```python
from build123d import *

# Parameters (mm, degrees)
SALIENTE_EXTRUIR1_DEPTH = 4
SALIENTE_EXTRUIR2_DEPTH = 30
SALIENTE_EXTRUIR5_DEPTH = 4
SALIENTE_EXTRUIR7_DEPTH = 4
CORTAR_EXTRUIR2_DEPTH   = 31
CROQUIS13_R             = 2.05
CORTAR_EXTRUIR3_DEPTH   = 4
CORTAR_EXTRUIR4_DEPTH   = 5
CORTAR_EXTRUIR5_DEPTH   = 2


with BuildPart() as part:
    # Croquis1 → Saliente-Extruir1 (new body)
    with BuildSketch(Plane(origin=(0, 0, 0), x_dir=(1, 0, 0), z_dir=(0, 1, 0))):
        Polygon((-11.66726189, 1.66726189), (11.66726189, -21.66726189), (11.66726189, 21.66726189), (-11.66726189, 21.66726189), align=None)
    extrude(amount=SALIENTE_EXTRUIR1_DEPTH)

    # Croquis3 → Saliente-Extruir2 (add)
    with BuildSketch(Plane.XZ):
        Polygon((-11.66726189, -1.66726189), (-11.66726189, 3.98959236), (11.66726189, 27.324116139), (11.66726189, 21.66726189), align=None)
    extrude(amount=-SALIENTE_EXTRUIR2_DEPTH)

    # Croquis7 → Saliente-Extruir5 (add)
    with BuildSketch(Plane(origin=(11.66726189, 0, 0), x_dir=(0, 0, -1), z_dir=(1, 0, 0))):
        Polygon((-21.66726189, 30), (21.66726189, 4), (21.66726189, 0), (-27.324116139, 0), (-27.324116139, 30), align=None)
    extrude(amount=SALIENTE_EXTRUIR5_DEPTH)

    # Croquis10 → Saliente-Extruir7 (add)
    with BuildSketch(Plane.ZY.offset(11.66726189)):
        Polygon((-1.66726189, 30), (-21.66726189, 4), (-21.66726189, 0), (3.98959236, 0), (3.98959236, 30), align=None)
    extrude(amount=SALIENTE_EXTRUIR7_DEPTH)

    # Croquis11 → Cortar-Extruir2 (cut, through all)
    with BuildSketch(Plane(origin=(0, 30, 0), x_dir=(1, 0, 0), z_dir=(0, 1, 0))):
        Polygon((-11.66726189, -3.98959236), (-15.66726189, 0.01040764), (-15.66726189, -3.98959236), align=None)
    extrude(amount=-CORTAR_EXTRUIR2_DEPTH, mode=Mode.SUBTRACT)

    # Croquis13 → Cortar-Extruir3 (cut)
    with BuildSketch(Plane(origin=(-7.828427125, 0, 7.828427125), x_dir=(0.707106781, 0, 0.707106781), z_dir=(-0.707106781, 0, 0.707106781))):
        with Locations((-3.428932188, 15.375)):
            Circle(CROQUIS13_R)
        with Locations((17.571067812, 15.375)):
            Circle(CROQUIS13_R)
    extrude(amount=-CORTAR_EXTRUIR3_DEPTH, mode=Mode.SUBTRACT)

    # Croquis14 → Cortar-Extruir4 (cut, through all)
    with BuildSketch(Plane(origin=(0, 4, 0), x_dir=(1, 0, 0), z_dir=(0, 1, 0))):
        with BuildLine():
            Line((-6, 17.644253814), (6, 17.644253814))
            ThreePointArc((6, 17.644253814), (8.1, 15.544253814), (6, 13.444253814))
            Line((6, 13.444253814), (-6, 13.444253814))
            ThreePointArc((-6, 13.444253814), (-8.1, 15.544253814), (-6, 17.644253814))
        make_face()
        with BuildLine():
            Line((-6, 7.644253814), (6, 7.644253814))
            ThreePointArc((6, 7.644253814), (8.1, 5.544253814), (6, 3.444253814))
            Line((6, 3.444253814), (-6, 3.444253814))
            ThreePointArc((-6, 3.444253814), (-8.1, 5.544253814), (-6, 7.644253814))
        make_face()
    extrude(amount=-CORTAR_EXTRUIR4_DEPTH, mode=Mode.SUBTRACT)

    # Croquis15 → Cortar-Extruir5 (cut)
    with BuildSketch(Plane(origin=(-5, 0, 5), x_dir=(-0.707106781, 0, -0.707106781), z_dir=(0.707106781, 0, -0.707106781))):
        Polygon((-13.587350954, 15.375), (-15.579209383, 18.825), (-19.562926241, 18.825), (-21.554784669, 15.375), (-19.562926241, 11.925), (-15.579209383, 11.925), align=None)
        Polygon((-0.554784669, 15.375), (1.437073759, 11.925), (5.420790617, 11.925), (7.412649046, 15.375), (5.420790617, 18.825), (1.437073759, 18.825), align=None)
    extrude(amount=-CORTAR_EXTRUIR5_DEPTH, mode=Mode.SUBTRACT)


solid = part.part
```
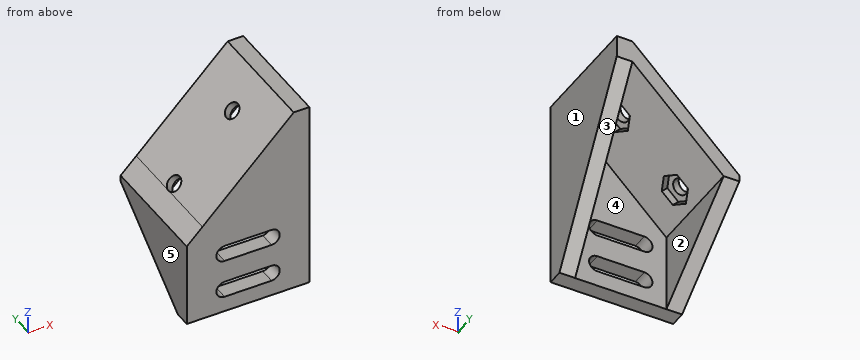
The model under review builds one solid part; all positions refer to its coordinate system, in mm. Face numbers are marked on the shaded views. A direction names the side the tool comes from. Round coordinates to 2 decimals unless told otherwise and drop trailing zeros. Loops run counter-clockwise (first coordinate to the right, second up) from the corner with the lowest first, then second, coordinate; pieces in that order, holes last. Notation, with made-up numbers: (-37, 83) - (-19, 83) arc R22 ccw to (-19, 111) - close; hole circle Ø9 at (79.25, 28). An arc over 180 degrees is marked (long way). Write each question's results on one line, items separated by ' | '. Start each with the question number.
Q1. Wall thickness on line 1 along X through (y, z) = (5.5, -17); line 2 along X through (y, z) = (17.5, 19.5); line 3 along X through (y, z) = (12, -8.5): over which ranges is each line inside the solid? List them lowest first. Write a range as [from, to].
Q2. Tool access review of the marked faces 4 and 5: name each direction out of +Z, -Z, +X, -X, +Y, -Y from which nothing blocks a thin tool from reaching the whole face with its end or side.
Q3. Insertion check: P1, Ø2, axis at x = -10.5, y = 8.5, coming from the +Z side; P2, Ø4.5, axis at x = -1.5, y = 1, coming from the +Z side; P3, Ø3, axis at y = 7.5, z = 13.5, coming from the -X side; P4, Ø3.5, axis at x = 7, z = 18, coming from the -Y side. Each pin has a flat end and moves straight along its axis. Give the tip position at first contact, or say it passes through.
Q4. Take a section at B-B on y = 23. Give the boundary of the cut face in (x, z), plus the area to 3 significant figures.
Q5. Draft analysis for pull direction X (two halves, no side actions). For the marked faces 1, 2 and 3, state which applies: pulls with the +X half, pulls with the -X half, needs draft (parallel to the pull), parting line crosses it, or undercut.
Q6. Take a section at A-A on z = -5. Give the boundary of the cut face in (x, y).
Data:
1) line 1: x = [-15.67, -11.67], [11.67, 15.67] | line 2: x = [3.84, 6.67], [9.25, 9.5], [11.67, 15.67] | line 3: x = [-15.67, -11.67]
2) face 4: -Z, +Y | face 5: +Z, -Z, -X, +Y, -Y
3) P1: stops at z = 6.16 | P2: stops at z = 16.41 | P3: stops at x = -3.66 | P4: stops at y = 0
4) outline: (-15.67, -7.05) - (-11.67, -7.05) - (-11.67, -1.67) - (11.67, 21.67) - (11.67, 10) - (15.67, 10) - (15.67, 27.32) - (11.67, 27.32) - (-15.67, -0.01) - close | area: 237 mm²
5) face 1: pulls with the +X half | face 2: undercut | face 3: needs draft
6) outline: (-15.67, 0) - (-8.03, 0) - (-8.03, 4) - (-11.67, 4) - (-11.67, 25.67) - (-15.67, 25.67) - close; (8.03, 0) - (15.67, 0) - (15.67, 14) - (11.67, 14) - (11.67, 4) - (8.03, 4) - close
